Source: CAD feature listing. Evaluate the final solid. Frame: model axes, mm. A direction names the side the tool comes from. Coordinates: 2 decimals unless noted, no trailing zeros. Loops run counter-clockwise (first coordinate to the right, second up) from the corner with the lowest first, then second, coordinate; pieces in that order, holes last. Notation, with made-up numbers: (81, 12.25) -> (126, 12.25) arc R32 cw to (126, 43.25) -> close; hole circle Ø7 at (12.5, 62). An arc over 180 degrees is marked (long way). Answer as a JSON object with one key per item and string values. Group by question number.
from build123d import *

# Parameters (mm, degrees)
SKETCH1_R                = 60
BOSS_EXTRUDE1_DEPTH      = 25.1
SKETCH3_R                = 47.5
CUT_EXTRUDE2_DEPTH       = 14
CUT_EXTRUDE5_DEPTH       = 89.487343728
CUT_EXTRUDE5_DEPTH_BACK  = 89.487343728
SKETCH2_R                = 2.494998654
SKETCH2_R_2              = 2.5
SKETCH2_R_3              = 2.444443829
SKETCH6_R                = 3
CUT_EXTRUDE6_DEPTH       = 6
CUT_EXTRUDE7_DEPTH       = 87
CUT_EXTRUDE7_DEPTH_BACK  = 87
BOSS_EXTRUDE2_DEPTH      = 30
BOSS_EXTRUDE2_DEPTH_BACK = 23
SKETCH8_W                = 24.8
SKETCH8_H                = 24.8
FILLET1_R                = 30
SKETCH9_R                = 6.1
CUT_EXTRUDE8_DEPTH       = 40
FILLET2_R                = 6
CUT_EXTRUDE9_DEPTH       = 3


with BuildPart() as part:
    # Sketch1 → Boss-Extrude1 (new body)
    with BuildSketch(Plane.XY):
        Circle(SKETCH1_R)
    extrude(amount=BOSS_EXTRUDE1_DEPTH)

    # Sketch3 → Cut-Extrude2 (cut)
    with BuildSketch(Plane.XY.offset(25.1)):
        Circle(SKETCH3_R)
    extrude(amount=-CUT_EXTRUDE2_DEPTH, mode=Mode.SUBTRACT)

    # Sketch2 → Cut-Extrude5 (cut, two sides: drawn at the far end of the back side and taken through both)
    with BuildSketch(Plane.XY.offset(25.1).offset(-CUT_EXTRUDE5_DEPTH_BACK)):
        with Locations((-16.664697145, -50.733104448)):
            Circle(SKETCH2_R)
        with Locations((-50.733105114, 16.664696544)):
            Circle(SKETCH2_R_2)
        with Locations((16.664695878, 50.733104512)):
            Circle(SKETCH2_R_3)
        with Locations((50.733103846, -16.66469648)):
            Circle(SKETCH2_R_2)
    extrude(amount=CUT_EXTRUDE5_DEPTH + CUT_EXTRUDE5_DEPTH_BACK, mode=Mode.SUBTRACT)

    # Sketch6 → Cut-Extrude6 (cut)
    with BuildSketch(Plane(origin=(0, 0, 0), x_dir=(-1, 0, 0), z_dir=(0, 0, -1))):
        with Locations((11.973502988, 47.212610548)):
            Circle(SKETCH6_R)
        with Locations((27.381285989, 40.029281029)):
            Circle(SKETCH6_R)
        with Locations((-19.717656658, -20.762902692)):
            Circle(SKETCH6_R)
        with Locations((-4.309873657, -27.946232212)):
            Circle(SKETCH6_R)
    extrude(amount=-CUT_EXTRUDE6_DEPTH, mode=Mode.SUBTRACT)

    # Sketch7 → Cut-Extrude7 (cut, two sides: drawn at the far end of the back side and taken through both)
    with BuildSketch(Plane.XY.offset(11.1).offset(-CUT_EXTRUDE7_DEPTH_BACK)):
        Polygon((-32.400942803, 32.871850778), (-3.10901045, -26.912408633), (24.254242539, -13.505492441), (-3.650778768, 46.958298756), align=None)
    extrude(amount=CUT_EXTRUDE7_DEPTH + CUT_EXTRUDE7_DEPTH_BACK, mode=Mode.SUBTRACT)

    # Sketch8 → Boss-Extrude2 (add, two sides: drawn at the far end of the back side and taken through both)
    with BuildSketch(Plane(origin=(33.53796733, -68.45033352, 0), x_dir=(-0.8980042769467113, -0.4399867254650012, 0), z_dir=(0.4399867254650012, -0.8980042769467113, 0)).offset(-BOSS_EXTRUDE2_DEPTH_BACK)):
        with Locations((-0.981202476, -12.478185074)):
            Rectangle(SKETCH8_W, SKETCH8_H)
    extrude(amount=BOSS_EXTRUDE2_DEPTH + BOSS_EXTRUDE2_DEPTH_BACK)

    # Fillet1
    fillet1_edges = [part.edges().sort_by_distance(p)[0] for p in [
        (37.75068654, -46.635669457, 12.478185074),
        (15.662587056, -57.91962851, 12.478185074),
    ]]
    fillet(fillet1_edges, radius=FILLET1_R)

    # Sketch9 → Cut-Extrude8 (cut)
    with BuildSketch(Plane(origin=(46.737569094, -95.390461829, 0), x_dir=(0.8980042769467111, 0.43998672546500134, 0), z_dir=(0.43998672546500134, -0.8980042769467111, 0))):
        with Locations((0.981202476, 12.478185074)):
            Circle(SKETCH9_R)
    extrude(amount=-CUT_EXTRUDE8_DEPTH, mode=Mode.SUBTRACT)

    # Fillet2
    # the kernel refuses this fillet: 6 mm, written as the material it takes off along each edge
    with BuildSketch(Plane(origin=(43.083240962, -113.884645314, 0.078185074), x_dir=(0.8980042769467113, 0.4399867254650012, 0), z_dir=(-0.43998672546500117, 0.8980042769467113, 0))) as fillet2_piece_1:
        with BuildLine():
            CenterArc((FILLET2_R, -FILLET2_R), FILLET2_R, 90, 90)
            Line((0, -FILLET2_R), (0, 0))
            Line((0, 0), (FILLET2_R, 0))
        make_face()
    extrude(amount=41.321991464, mode=Mode.SUBTRACT)
    with BuildSketch(Plane(origin=(43.083240962, -113.884645314, 24.878185074), x_dir=(0.8980042769467111, 0.4399867254650013, 0), z_dir=(-0.4399867254650013, 0.8980042769467113, 0))) as fillet2_piece_2:
        with BuildLine():
            CenterArc((FILLET2_R, FILLET2_R), FILLET2_R, 180, 90)
            Line((0, FILLET2_R), (0, 0))
            Line((0, 0), (FILLET2_R, 0))
        make_face()
    extrude(amount=41.321991464, mode=Mode.SUBTRACT)
    with BuildSketch(Plane(origin=(46.711419385, -64.924349442, 24.878185074), x_dir=(-0.8980042769467113, -0.4399867254650012, 0), z_dir=(0.4399867254650012, -0.8980042769467113, 0))) as fillet2_piece_3:
        with BuildLine():
            CenterArc((FILLET2_R, FILLET2_R), FILLET2_R, 180, 90)
            Line((0, FILLET2_R), (0, 0))
            Line((0, 0), (FILLET2_R, 0))
        make_face()
    extrude(amount=42.37020475, mode=Mode.SUBTRACT)
    with BuildSketch(Plane(origin=(46.711419385, -64.924349442, 0.078185074), x_dir=(-0.8980042769467113, -0.4399867254650012, 0), z_dir=(0.43998672546500117, -0.8980042769467113, 0))) as fillet2_piece_4:
        with BuildLine():
            CenterArc((FILLET2_R, -FILLET2_R), FILLET2_R, 90, 90)
            Line((0, -FILLET2_R), (0, 0))
            Line((0, 0), (FILLET2_R, 0))
        make_face()
    extrude(amount=42.37020475, mode=Mode.SUBTRACT)
    with BuildSketch(Plane(origin=(-2.03801506, -89.976922011, 24.878185074), x_dir=(-0.45951638072731243, 0.8881692945848058, 0), z_dir=(-0.8881692945848058, -0.45951638072731243, 0))) as fillet2_piece_5_section:
        with BuildLine():
            CenterArc((30 + FILLET2_R, FILLET2_R), FILLET2_R, 180, 90)
            Line((30, FILLET2_R), (30, 0))
            Line((30, 0), (30 + FILLET2_R, 0))
        make_face()
    fillet2_piece_5 = revolve(axis=Axis((-2.03801506, -89.976922011, 24.878185074), (0, 0, -1)), revolution_arc=91.252870665, mode=Mode.PRIVATE)
    fillet2_piece_5 = fillet2_piece_5 - Plane(origin=(0, 0, 24.878185074), x_dir=(1, 0, 0), z_dir=(0, 0, -1)) * Cylinder(60, 144, mode=Mode.PRIVATE)
    add(fillet2_piece_5, mode=Mode.SUBTRACT)
    with BuildSketch(Plane(origin=(-2.03801506, -89.976922011, 0.078185074), x_dir=(-0.45951638072731255, 0.8881692945848058, 0), z_dir=(-0.8881692945848058, -0.45951638072731255, 0))) as fillet2_piece_6_section:
        with BuildLine():
            CenterArc((30 + FILLET2_R, -FILLET2_R), FILLET2_R, 90, 90)
            Line((30 + FILLET2_R, 0), (30, 0))
            Line((30, 0), (30, -FILLET2_R))
        make_face()
    fillet2_piece_6 = revolve(axis=Axis((-2.03801506, -89.976922011, 0.078185074), (0, 0, -1)), revolution_arc=91.252870665, mode=Mode.PRIVATE)
    fillet2_piece_6 = fillet2_piece_6 - Plane(origin=(0, 0, 0.078185074), x_dir=(1, 0, 0), z_dir=(0, 0, -1)) * Cylinder(60, 144, mode=Mode.PRIVATE)
    add(fillet2_piece_6, mode=Mode.SUBTRACT)
    with BuildSketch(Plane(origin=(73.651547694, -51.724747678, 0.078185074), x_dir=(-0.44255176351936526, 0.8967429601652304, 0), z_dir=(0.8967429601652304, 0.44255176351936526, 0))) as fillet2_piece_7_section:
        with BuildLine():
            CenterArc((30 + FILLET2_R, FILLET2_R), FILLET2_R, 180, 90)
            Line((30 + FILLET2_R, 0), (30, 0))
            Line((30, 0), (30, FILLET2_R))
        make_face()
    fillet2_piece_7 = revolve(axis=Axis((73.651547694, -51.724747678, 0.078185074), (0, 0, 1)), revolution_arc=89.836226794, mode=Mode.PRIVATE)
    fillet2_piece_7 = fillet2_piece_7 - Plane(origin=(0, 0, 0.078185074), x_dir=(1, 0, 0), z_dir=(0, 0, -1)) * Cylinder(60, 144, mode=Mode.PRIVATE)
    add(fillet2_piece_7, mode=Mode.SUBTRACT)
    with BuildSketch(Plane(origin=(73.651547694, -51.724747678, 24.878185074), x_dir=(-0.44255176351936476, 0.8967429601652306, 0), z_dir=(0.8967429601652306, 0.44255176351936476, 0))) as fillet2_piece_8_section:
        with BuildLine():
            CenterArc((30 + FILLET2_R, -FILLET2_R), FILLET2_R, 90, 90)
            Line((30 + FILLET2_R, 0), (30, 0))
            Line((30, 0), (30, -FILLET2_R))
        make_face()
    fillet2_piece_8 = revolve(axis=Axis((73.651547694, -51.724747678, 24.878185074), (0, 0, 1)), revolution_arc=89.836226794, mode=Mode.PRIVATE)
    fillet2_piece_8 = fillet2_piece_8 - Plane(origin=(0, 0, 24.878185074), x_dir=(1, 0, 0), z_dir=(0, 0, -1)) * Cylinder(60, 144, mode=Mode.PRIVATE)
    add(fillet2_piece_8, mode=Mode.SUBTRACT)

    # Sketch12 → Cut-Extrude9 (cut)
    with BuildSketch(Plane(origin=(0, 0, 0), x_dir=(-1, 0, 0), z_dir=(0, 0, -1))):
        Polygon((16.569778792, 40.628497592), (19.583965842, 46.780394242), (22.182787305, 45.507074086), (19.168600256, 39.355177436), align=None)
        Polygon((-11.458078278, -19.775108918), (-14.390783054, -26.33846158), (-12.052056845, -27.383475291), (-9.156328603, -20.902875599), align=None)
    extrude(amount=-CUT_EXTRUDE9_DEPTH, mode=Mode.SUBTRACT)


solid = part.part
1. Reachability of faces 1 (the face through (20, 1, 11.1)), 2 (the face through (4, -28, 6)), 3 (the face through (-17.96, 3.4, 5.47)) from +Z, -Z, +X, -X, +Y, -Y: full face, straight path, thin tool, end or side. Return the list, or none.
2. Pin query (flat end, axial travel): pin 1 Ø2 at (y, z) = (19, 4) entering from -X; pin 2 Ø8 at (x, y) = (34.5, 14) entering from -Z; pin 3 Ø12 at (y, z) = (43, 10) entering from +X; pin 4 Ø6 at (y, z) = (-18.5, 21) entering from -X. Return the tip coordinate at first contact, or that it passes through.
3. Section query A-A on y = 0. Return loops of the section in (x, z).
4. Section query B-B on z = 21.5. Return loops of the section in (x, y) (3 decimals), then the cut area to 3 significant figures.
5. Ray query, L1, parallel to Y at x = -30, z = 2.25; L2, parallel to Y at x = 16, z = 22.25; L3, parallel to Z at x = 24, y = 40.5. Return the intervals inside material, ascending.
6. Mould query, pull axis X, two halves, no side actions, for faces 4 (the face through (32.31, -88.009, 23.074)), 5 (the face through (17.979, 52.794, 12.374)), 6 (the face through (-11.323, 44.284, 2.958)), 7 (the face through (43.727, -49.601, 12.389)). Classes: pulls with the +X half, pulls with the -X half, needs draft (parallel to the pull), parting line crosses it, or undercut.
Solved:
{
 "1": {"face 1": "+Z", "face 2": "-Z", "face 3": "+Z, -Z"},
 "2": {"pin 1": "x = -57.24", "pin 2": "z = 0", "pin 3": "x = 47.23", "pin 4": "x = -57.96"},
 "3": {"outline": "(-60, 0) -> (-16.3, 0) -> (-16.3, 11.1) -> (-47.5, 11.1) -> (-47.5, 25.1) -> (-60, 25.1) -> close; (18.02, 0) -> (60, 0) -> (60, 25.1) -> (47.5, 25.1) -> (47.5, 11.1) -> (18.02, 11.1) -> close"},
 "4": {"outline": "(3.577, -59.893) arc R30.603 cw to (25.444, -76.512) -> (37.025, -100.149) -> (58.212, -89.768) -> (46.17, -65.19) arc R30.603 cw to (46.1, -38.403) arc R60 ccw (long way) to start; hole circle Ø5 at (-50.733, 16.665); hole circle Ø95 at (0, 0); hole circle Ø4.99 at (-16.665, -50.733); hole circle Ø4.889 at (16.665, 50.733); hole circle Ø5 at (50.733, -16.665)", "area": "5,370 mm^2"},
 "5": {"L1": "-51.96 to 27.97, 34.05 to 38.57, 41.49 to 51.96", "L2": "-64.72 to -44.72, 44.72 to 48.38, 53.09 to 57.83", "L3": "0 to 11.1"},
 "6": {"face 4": "pulls with the -X half", "face 5": "undercut", "face 6": "undercut", "face 7": "pulls with the +X half"}
}
